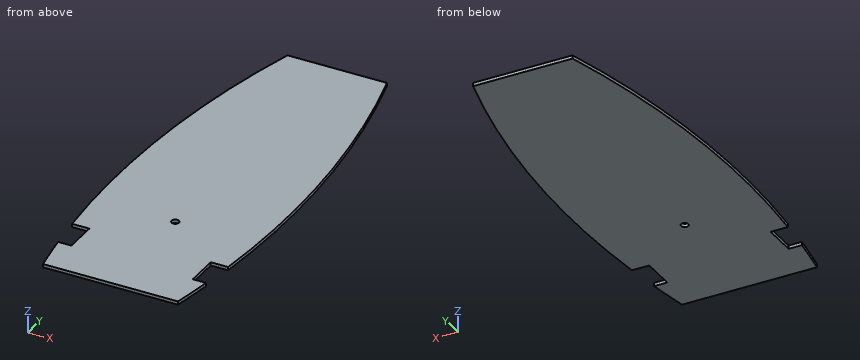
```python
from build123d import *

# Parameters (mm, degrees)
BOSS_EXTRUDE1_DEPTH = 5
SKETCH3_R           = 5.5
CUT_EXTRUDE1_DEPTH  = 1008.818415992
SKETCH4_W           = 203.352119636
SKETCH4_H           = 409.958390473
CUT_EXTRUDE2_DEPTH  = 1008.818415992


with BuildPart() as part:
    # Sketch2 → Boss-Extrude1 (new body)
    with BuildSketch(Plane.XY):
        with BuildLine():
            Line((-75, 0), (75, 0))
            ThreePointArc((75, 0), (125.183748831, -378.01295639), (72.466338168, -755.680903745))
            Line((72.466338168, -755.680903745), (4.813443083, -996.353057902))
            ThreePointArc((4.813443083, -996.353057902), (3.01949586, -998.985303596), (0, -1000))
            ThreePointArc((0, -1000), (-3.01949586, -998.985303596), (-4.813443083, -996.353057902))
            Line((-4.813443083, -996.353057902), (-72.466338168, -755.680903745))
            ThreePointArc((-72.466338168, -755.680903745), (-125.183748831, -378.01295639), (-75, 0))
        make_face()
    extrude(amount=BOSS_EXTRUDE1_DEPTH)

    # Sketch3 → Cut-Extrude1 (cut, through all)
    with BuildSketch(Plane(origin=(0, 0, 0), x_dir=(-1, 0, 0), z_dir=(0, 0, -1))):
        with Locations((0, -450)):
            Circle(SKETCH3_R)
    extrude(amount=-CUT_EXTRUDE1_DEPTH, mode=Mode.SUBTRACT)

    # Sketch4 → Cut-Extrude2 (cut, through all)
    with BuildSketch(Plane(origin=(0, 0, 0), x_dir=(-1, 0, 0), z_dir=(0, 0, -1))):
        with BuildLine():
            Line((-117.553772729, -520), (-91.431313106, -520))
            Line((-91.431313106, -520), (-91.431313106, -570))
            Line((-91.431313106, -570), (-111.431313106, -570))
            ThreePointArc((-111.431313106, -570), (-125.443374502, -546.340920484), (-117.553772729, -520))
        make_face()
        with BuildLine():
            Line((117.553772729, -520), (91.431313106, -520))
            Line((91.431313106, -520), (91.431313106, -570))
            Line((91.431313106, -570), (111.431313106, -570))
            ThreePointArc((111.431313106, -570), (125.443374502, -546.340920484), (117.553772729, -520))
        make_face()
        with Locations((0, -834.979195237)):
            Rectangle(SKETCH4_W, SKETCH4_H)
    extrude(amount=-CUT_EXTRUDE2_DEPTH, mode=Mode.SUBTRACT)


solid = part.part
```
Verification items for the finished model (mm, model axes). Give positions to 0.01 mm unless a question says otherwise; leave off trailing zeros. Loops run counter-clockwise (first coordinate to the right, second up) from the corner with the lowest first, then second, coordinate; pieces in that order, holes last.
1. Thickness scan on line 1 (Y direction, x = 0, z = 1); line 2 (X direction, y = -450, z = 3.3); line 3 (X direction, y = -514, z = 4.1). Record the ranges inside material, lowest first.
2. Section check D-D, the plane y = -60.5. Enter the section's corners in (x, z).
3. Section check B-B, the plane x = 0. Enter the section's corners in (y, z).
4. Section check C-C, the plane y = -450. Enter the section's corners in (x, z).
5. Section check A-A, the plane z = 0.9. Enter the section's corners in (x, y), then the cut area to 3 significant figures.
Geometry says:
1. line 1: y = -630 to -455.5, -444.5 to 0
1. line 2: x = -123.11 to -5.5, 5.5 to 123.11
1. line 3: x = -118.17 to 118.17
2. outline: (-90.14, 0) - (90.14, 0) - (90.14, 5) - (-90.14, 5) - close
3. outline: (-630, 0) - (-455.5, 0) - (-455.5, 5) - (-630, 5) - close; (-444.5, 0) - (0, 0) - (0, 5) - (-444.5, 5) - close
4. outline: (-123.11, 0) - (-5.5, 0) - (-5.5, 5) - (-123.11, 5) - close; (5.5, 0) - (123.11, 0) - (123.11, 5) - (5.5, 5) - close
5. outline: (-117.55, -520) - (-91.43, -520) - (-91.43, -570) - (-111.43, -570) arc R1413.12 ccw to (-101.68, -630) - (101.68, -630) arc R1413.12 ccw to (111.43, -570) - (91.43, -570) - (91.43, -520) - (117.55, -520) arc R1413.12 ccw to (75, 0) - (-75, 0) arc R1413.12 ccw to start; hole circle Ø11 at (0, -450)
5. area: 139,000 mm2
